Read the model definition and answer for the solid it produces. Units are mm, in the model's axes. Coordinates: 2 decimals unless noted, no trailing zeros. Write each loop counter-clockwise with the first axis right and the second up, starting at its lowest first coordinate (ties: lowest second). Pieces come first, ordered by that corner, then holes.
(1) The part is cut by section A-A, the plane z = 1.6. Determine the outline of the cut face in (x, y).
(2) A straight line is drawn through the part: line 1 along Y through (x, z) = (4.25, 2.5). Find the intervals that lie inside material, in ascending order.
(3) Given pin 1 (1.5 mm diameter, centred on y = 92.5, z = 2, fed in from -X); pin 2 (1 mm diameter, centred on x = 4, z = 1, fed in from -Y); pin 3 (1.5 mm diameter, centred on y = -92.5, z = 2, fed in from +X), each flat-ended and moving along its own axis, determine where each tip first touches the part or whether it passes through.
(4) The part is cut by section B-B, the plane x = -8. Determine the outline of the cut face in (y, z).
Autodesk Inventor part; units mm, degrees
ref_plane "YZ Plane" through (0, 0, 0) normal (1, 0, 0) x (0, 1, 0)
ref_plane "XZ Plane" through (0, 0, 0) normal (0, 1, 0) x (-1, 0, 0)
ref_plane "XY Plane" through (0, 0, 0) normal (0, 0, 1) x (1, 0, 0)
sketch "Sketch1" plane through (0, 0, 0) normal (0, 0, 1) x (1, 0, 0)
  line L0 (5, -90.5) -> (5, 90.5)
  line L1 (-5, -90.5) -> (5, 90.5) construction
  line L2 (5, -90.5) -> (-5, 90.5) construction
  line L3 (3, 90.5) -> (3, 93.5)
  line L4 (3, 93.5) -> (-3, 93.5)
  line L5 (-3, 93.5) -> (-3, 90.5)
  line L6 (5, 90.5) -> (3, 90.5)
  line L7 (-3, 90.5) -> (-5, 90.5)
  line L8 (3, -90.5) -> (3, -93.5)
  line L9 (3, -93.5) -> (-3, -93.5)
  line L10 (-3, -93.5) -> (-3, -90.5)
  line L11 (-5, -90.5) -> (-3, -90.5)
  line L12 (3, -90.5) -> (5, -90.5)
  line L13 (-5, -90.5) -> (-10, -90.5)
  line L14 (-10, -90.5) -> (-10, 90.5)
  line L15 (-10, 90.5) -> (-5, 90.5)
  point P0 (0, 0)
  dimension "d0" = 10
  dimension "d1" = 181
  dimension "d2" = 6
  dimension "d3" = 3
  dimension "d5" = 6
  dimension "d6" = 3
  dimension "d8" = 3.162
  dimension "d9" = 3.162
  dimension "d12" = 5
  dimension "d13" = 90
  dimension "d14" = 2
  dimension "d15" = 15
  dimension "d16" = 3
extrude "Extrusion1" add sketch "Sketch1" along normal blind 3
equation "\"BendRadius\" = Thickness"
equation "\"BendReliefWidth\" = Thickness"
equation "\"BendReliefDepth\" = 0.5 * Thickness"
equation "\"CornerReliefSize\" = 4 * Thickness"
equation "\"MinimumRemnant\" = 2 * Thickness"
equation "\"TransitionRadius\" = BendRadius"
equation "\"JacobiRadiusSize\" = BendRadius"
equation "\"GapSize\" = Thickness"
properties part number "3 binnen dunne cover plaat"
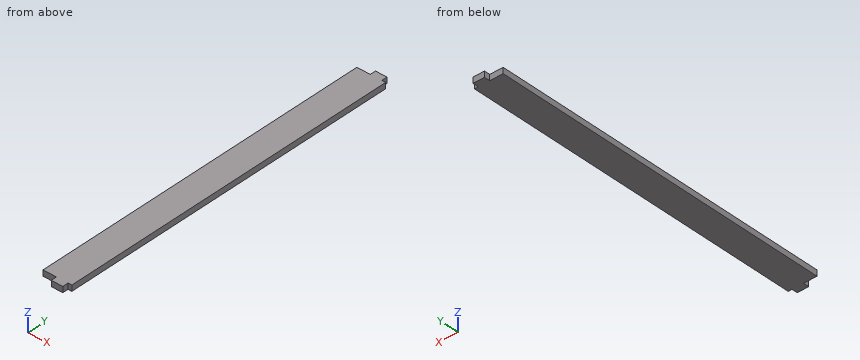
Computed:
1. outline: (-10, -90.5) - (-3, -90.5) - (-3, -93.5) - (3, -93.5) - (3, -90.5) - (5, -90.5) - (5, 90.5) - (3, 90.5) - (3, 93.5) - (-3, 93.5) - (-3, 90.5) - (-10, 90.5) - close
2. line 1: y = -90.5 to 90.5
3. pin 1: stops at x = -3
3. pin 2: stops at y = -90.5
3. pin 3: stops at x = 3
4. outline: (-90.5, 0) - (90.5, 0) - (90.5, 3) - (-90.5, 3) - close
